Input: dimensioned drawing with shaded views. Units: mm. Origin: part minimum x, y, z. A direction names the side the tool comes from. Coordinates: 2 decimals unless noted, no trailing zeros. Write each loop counter-clockwise with the first axis right and the second up, starting at its lowest first coordinate (ties: lowest second). Pieces come first, ordered by that corner, then holes. Notation, with made-up numbers: M -21.75,-4.5 L 5.25,-4.5 A25 ccw 5.25,19.5 Z; hole C -30,-32 d5. An arc over 180 degrees is marked long. Use one line per item in the form item = value.
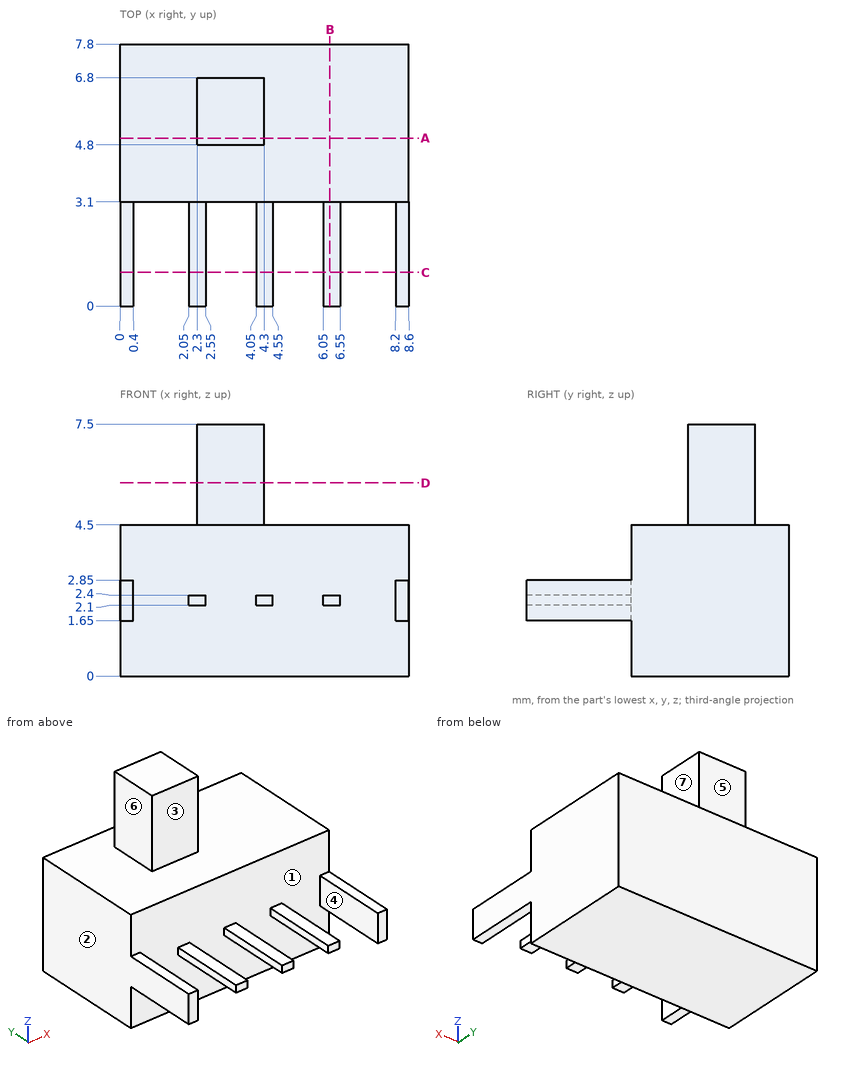
(1) Section query C-C on y = 1. Return the cut outline in (x, z), plus the area to 3 significant figures.
Computed:
outline = M 0,1.65 L 0.4,1.65 L 0.4,2.85 L 0,2.85 Z; M 2.05,2.1 L 2.55,2.1 L 2.55,2.4 L 2.05,2.4 Z; M 4.05,2.1 L 4.55,2.1 L 4.55,2.4 L 4.05,2.4 Z; M 6.05,2.1 L 6.55,2.1 L 6.55,2.4 L 6.05,2.4 Z; M 8.2,1.65 L 8.6,1.65 L 8.6,2.85 L 8.2,2.85 Z
area = 1.41 mm^2
(2) Section query A-A on y = 5. Return the cut outline in (x, z).
Computed:
outline = M 0,0 L 8.6,0 L 8.6,4.5 L 4.3,4.5 L 4.3,7.5 L 2.3,7.5 L 2.3,4.5 L 0,4.5 Z
(3) First-contact query: pin 1 Ø1.4 at (x, y) = (6.5, 6.5) entering from +Z; pin 2 Ø1 at (y, z) = (7, 6) entering from +X; pin 3 Ø2 at (x, z) = (3, 6) entering from +Y. Flat tips, straight axial feed; report the tip coordinate or a pass-through.
Computed:
pin_1 = 4.5
pin_2 = 4.3
pin_3 = 6.8
(4) Set-up query: the marked faces 4, 5, 6 and 7. Return all of +Z, -Z, +X, -X, +Y, -Y with unobstructed straight access to the full face (end or side cutting, diameter ignored); none if empty.
Computed:
face_4 = +Z, -Z, -Y
face_5 = +Z, +X, -X, +Y
face_6 = +Z, -X, +Y, -Y
face_7 = +Z, +X, +Y, -Y
(5) Pull-direction query (X, two-part tool) for the marked faces 1, 2 and 3; classes: pulls with the +X half, pulls with the -X half, needs draft (parallel to the pull), parting line crosses it, or undercut.
Computed:
face_1 = undercut
face_2 = pulls with the -X half
face_3 = needs draft
(6) Section query B-B on x = 6.25. Return the cut outline in (y, z).
Computed:
outline = M 0,2.1 L 3.1,2.1 L 3.1,0 L 7.8,0 L 7.8,4.5 L 3.1,4.5 L 3.1,2.4 L 0,2.4 Z
(7) Section query D-D on z = 5.75. Return the cut outline in (x, y), plus the area to 3 significant figures.
Computed:
outline = M 2.3,4.8 L 4.3,4.8 L 4.3,6.8 L 2.3,6.8 Z
area = 4.00 mm^2
(8) Line query: probe 1 along Y at (x, z) = (2, 2.25); probe 2 along X at (y, z) = (3, 2.75); probe 3 along Z at (x, y) = (7.5, 4.5). Output: solid intervals per line, ascending.
Computed:
probe_1 = 3.1 to 7.8
probe_2 = 0 to 0.4, 8.2 to 8.6
probe_3 = 0 to 4.5
